from build123d import *

# Parameters (mm, degrees)
F0_R     = 9.25
F1_DEPTH = 64


with BuildPart() as f1:
    # F0 (on Top) → F1 (new body)
    with BuildSketch(Plane.XY):
        with BuildLine():
            Line((6.206515, 10.75), (-6.206515, 10.75))
            Line((-6.206515, 10.75), (-12.413031, 0))
            Line((-12.413031, 0), (-6.206515, -10.75))
            Line((-6.206515, -10.75), (6.206515, -10.75))
            Line((6.206515, -10.75), (11.581515, -1.440227))
            ThreePointArc((11.581515, -1.440227), (10.75, 0), (11.581515, 1.440227))
            Line((11.581515, 1.440227), (6.206515, 10.75))
        make_face()
        Circle(F0_R, mode=Mode.SUBTRACT)
        with BuildLine():
            Line((12.413031, 21.5), (6.206515, 10.75))
            Line((6.206515, 10.75), (11.581515, 1.440227))
            ThreePointArc((11.581515, 1.440227), (13.244546, 1.440227), (14.076062, 0))
            Line((14.076062, 0), (24.826062, 0))
            Line((24.826062, 0), (31.032577, 10.75))
            Line((31.032577, 10.75), (24.826062, 21.5))
            Line((24.826062, 21.5), (12.413031, 21.5))
        make_face()
        with Locations((18.619546, 10.75)):
            Circle(F0_R, mode=Mode.SUBTRACT)
        with BuildLine():
            Line((24.826062, 0), (14.076062, 0))
            ThreePointArc((14.076062, 0), (13.244546, -1.440227), (11.581515, -1.440227))
            Line((11.581515, -1.440227), (6.206515, -10.75))
            Line((6.206515, -10.75), (12.413031, -21.5))
            Line((12.413031, -21.5), (24.826062, -21.5))
            Line((24.826062, -21.5), (31.032577, -10.75))
            Line((31.032577, -10.75), (24.826062, 0))
        make_face()
        with Locations((18.619546, -10.75)):
            Circle(F0_R, mode=Mode.SUBTRACT)
    extrude(amount=F1_DEPTH)


solid = f1.part
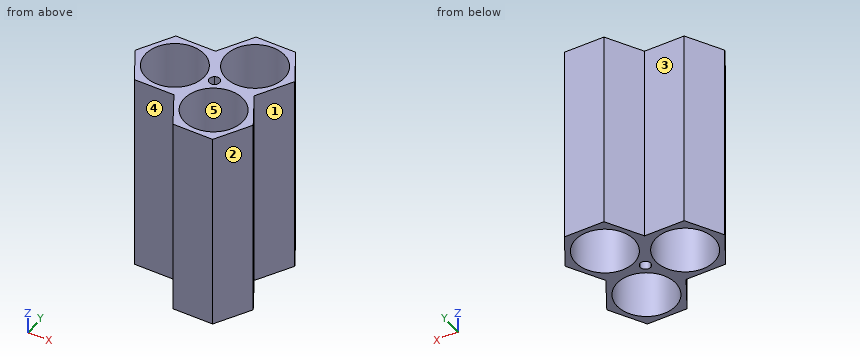
Geometry: final body of the model. Coordinates: model frame, mm. Face numbers are marked on the shaded views. A direction names the side the tool comes from. Coordinates: 2 decimals unless noted, no trailing zeros. Loops run counter-clockwise (first coordinate to the right, second up) from the corner with the lowest first, then second, coordinate; pieces in that order, holes last. Notation, with made-up numbers: M -10,-21.75 L 28,-21.75 A24 ccw 28,6.25 Z; hole C 70,21 d6. An arc over 180 degrees is marked long. One line per item, written item: value. Start each with the question number.
1) Cut plane D-D (x = -8). Return loops of the section in (y, z).
2) Pin query (flat end, axial travel): P1, Ø8, axis at y = -6, z = 35.5, coming from the +X side; P2, Ø13.5, axis at x = 1, z = 27, coming from the +Y side; P3, Ø10, axis at y = 15, z = 29, coming from the +X side; P4, Ø15, axis at x = 18.62, y = 10.75, coming from the -Z side. Return the tip coordinate at first contact, or that it passes through.
3) Reachability of the marked faces 1, 2, 3, 4 and 5 from +Z, -Z, +X, -X, +Y, -Y: full face, straight path, thin tool, end or side. Return the list, or none.
4) Cut plane A-A (x = 0). Return loops of the section in (y, z), then the cut area to 3 significant figures.
5) Cut plane B-B (y = 4). Return loops of the section in (x, z) (3 decimals), then the cut area to 3 significant figures.
6) Material intervals for L1, parallel to X at y = -4, z = 52 (3 decimals); L2, parallel to Y at x = 11, z = 10.5; L3, parallel to Y at x = 0, z = 49, sorted ascending. Write a range as from..to.
7) Cut plane C-C (z = 19). Return loops of the section in (x, y), then the cut area to 3 significant figures.
Evaluation:
1. outline: M -7.64,0 L -4.64,0 L -4.64,64 L -7.64,64 Z; M 4.64,0 L 7.64,0 L 7.64,64 L 4.64,64 Z
2. P1: x = 30.6
2. P2: y = 13.42
2. P3: x = 31.03
2. P4: through
3. face 1: +Z, -Z, +X
3. face 2: +Z, -Z, +X, -Y
3. face 3: +Z, -Z, -X, +Y
3. face 4: +Z, -Z, -X, -Y
3. face 5: +Z, -Z
4. outline: M -10.75,0 L -9.25,0 L -9.25,64 L -10.75,64 Z; M 9.25,0 L 10.75,0 L 10.75,64 L 9.25,64 Z
4. area: 192 mm^2
5. outline: M -10.104,0 L -8.34,0 L -8.34,64 L -10.104,64 Z; M 8.34,0 L 12.295,0 L 12.295,64 L 8.34,64 Z; M 24.944,0 L 27.135,0 L 27.135,64 L 24.944,64 Z
5. area: 506 mm^2
6. L1: -10.104..-8.34, 8.34..12.295, 24.944..27.135
6. L2: -19.05..-15.99, -5.51..-0.88, 0.88..5.51, 15.99..19.05
6. L3: -10.75..-9.25, 9.25..10.75
7. outline: M -12.41,0 L -6.21,-10.75 L 6.21,-10.75 L 12.41,-21.5 L 24.83,-21.5 L 31.03,-10.75 L 24.83,0 L 31.03,10.75 L 24.83,21.5 L 12.41,21.5 L 6.21,10.75 L -6.21,10.75 Z; hole C 0,0 d18.5; hole C 18.62,-10.75 d18.5; hole C 18.62,10.75 d18.5; hole M 11.58,1.44 A1.66 ccw long 14.08,0 A1.66 ccw Z
7. area: 386 mm^2
